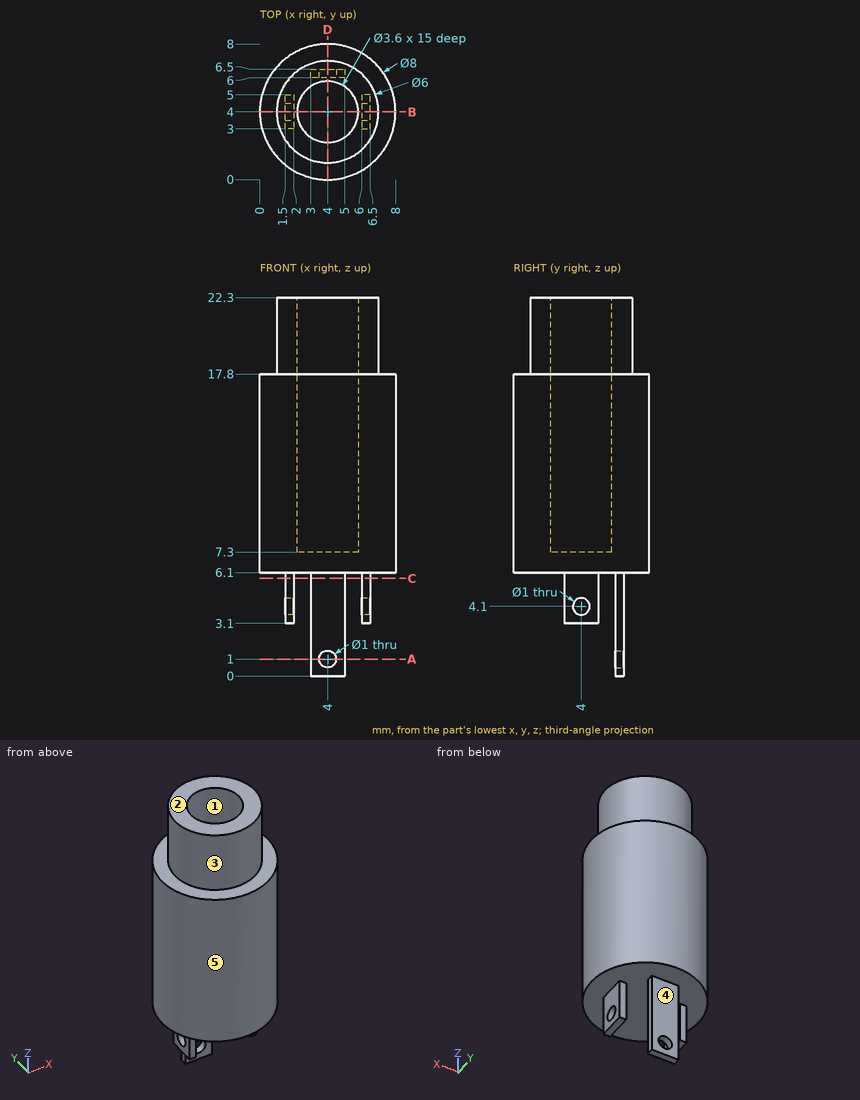
Print and shaded views of the part. All mm, measured from the part's lowest x, y and z. A direction names the side the tool comes from. Give positions to 0.01 mm unless a question says otherwise; leave off trailing zeros. Order: outer loops, then holes, each group sorted by start corner. A loop starts at its lowest first (then second) coordinate and runs counter-clockwise, first axis right, second up. Notation, with made-up numbers: (3, -39.5) - (56, -39.5) arc R11 ccw to (56, -27.5) - close; hole circle Ø8 at (21.5, 83). An arc over 180 degrees is marked (long way). Use a Markdown table: item, result.
1) Two-plate mould, pull along Y, no slides. Class the marked faces 1, 2 and 3: +Y half, -Y half, draft (parallel to the pull), parting line (faces both ways), or undercut.
Checked values:
| item | result |
|---|---|
| face 1 | undercut |
| face 2 | draft |
| face 3 | parting line |
2) Saw through at D-D on x = 4. List the corners of the cut face in (y, z).
Checked values:
| item | result |
|---|---|
| outline | (0, 6.1) - (6, 6.1) - (6, 1.5) - (6.5, 1.5) - (6.5, 6.1) - (8, 6.1) - (8, 17.8) - (7, 17.8) - (7, 22.3) - (5.8, 22.3) - (5.8, 7.3) - (2.2, 7.3) - (2.2, 22.3) - (1, 22.3) - (1, 17.8) - (0, 17.8) - close; (6, 0) - (6.5, 0) - (6.5, 0.5) - (6, 0.5) - close |
3) Saw through at A-A on z = 1. List the corners of the cut face in (x, y), plus the area to 3 significant figures.
Checked values:
| item | result |
|---|---|
| outline | (3, 6) - (3.5, 6) - (3.5, 6.5) - (3, 6.5) - close; (4.5, 6) - (5, 6) - (5, 6.5) - (4.5, 6.5) - close |
| area | 0.500 mm² |
4) Saw through at C-C on z = 5.75. List the corners of the cut face in (x, y), plus the area to 3 significant figures.
Checked values:
| item | result |
|---|---|
| outline | (1.5, 3) - (2, 3) - (2, 5) - (1.5, 5) - close; (3, 6) - (5, 6) - (5, 6.5) - (3, 6.5) - close; (6, 3) - (6.5, 3) - (6.5, 5) - (6, 5) - close |
| area | 3.00 mm² |
5) Saw through at B-B on y = 4. List the corners of the cut face in (x, z).
Checked values:
| item | result |
|---|---|
| outline | (0, 6.1) - (1.5, 6.1) - (1.5, 4.6) - (2, 4.6) - (2, 6.1) - (6, 6.1) - (6, 4.6) - (6.5, 4.6) - (6.5, 6.1) - (8, 6.1) - (8, 17.8) - (7, 17.8) - (7, 22.3) - (5.8, 22.3) - (5.8, 7.3) - (2.2, 7.3) - (2.2, 22.3) - (1, 22.3) - (1, 17.8) - (0, 17.8) - close; (1.5, 3.1) - (2, 3.1) - (2, 3.6) - (1.5, 3.6) - close; (6, 3.1) - (6.5, 3.1) - (6.5, 3.6) - (6, 3.6) - close |
6) Probe L1, parallel to Y at x = 1.95, z = 4.1; L2, parallel to X at y = 4.75, z = 3.75; L3, parallel to Z at x = 4, y = 6.2. List the from-to ranges inside material, lowest first. Write a range as from..to.
Checked values:
| item | result |
|---|---|
| L1 | 3..3.5, 4.5..5 |
| L2 | 1.5..2, 6..6.5 |
| L3 | 0..0.5, 1.5..22.3 |
7) 3-axis set-ups, long thin cutter, end or side, ignore diameter. For the marked faces 4 and 5: which of +Z, -Z, +X, -X, +Y, -Y reach the whole face in a straight line?
Checked values:
| item | result |
|---|---|
| face 4 | -Z, +X, -X, +Y |
| face 5 | +Z, -Z |
8) Flat gauge pins, fed straight in: P1, Ø2, axis at x = 5.5, z = 12, coming from the +Y side; P2, Ø4, axis at x = 1, y = 5, coming from the -Z side; P3, Ø2, axis at y = 4.5, z = 4, coming from the -X side. Where does each tip first touch, or does it go through?
Checked values:
| item | result |
|---|---|
| P1 | y = 7.97 |
| P2 | z = 3.1 |
| P3 | x = 1.5 |
